from build123d import *

# Parameters (mm, degrees)
SKETCH_1_W          = 6.3
SKETCH_1_H          = 11.9
SKETCH_1_W_2        = 3
SKETCH_1_H_2        = 1.2
EXTRUDE_2_DEPTH     = 3
SKETCH_7_W          = 6.3
SKETCH_7_H          = 5.7
EXTRUDE_4_DEPTH     = 2.8
SKETCH_8_W          = 6.3
SKETCH_8_H          = 6.2
EXTRUDE_5_DEPTH     = 5.2
SKETCH_5_R          = 2.7
SKETCH_5_R_2        = 2.95
CUT_EXTRUDE_3_DEPTH = 15.790960077
FILLET_1_R          = 3


with BuildPart() as part:
    # ｽｹｯﾁ1 → ﾎﾞｽ - 押し出し2 (new body)
    with BuildSketch(Plane.YZ):
        with Locations((0, 5.95)):
            Rectangle(SKETCH_1_W, SKETCH_1_H)
        with Locations((0, -0.6)):
            Rectangle(SKETCH_1_W_2, SKETCH_1_H_2)
    extrude(amount=-EXTRUDE_2_DEPTH)

    # ｽｹｯﾁ7 → ﾎﾞｽ - 押し出し4 (add)
    with BuildSketch(Plane(origin=(-3, 0, 0), x_dir=(0, -1, 0), z_dir=(-1, 0, 0))):
        with Locations((0, 2.85)):
            Rectangle(SKETCH_7_W, SKETCH_7_H)
    extrude(amount=EXTRUDE_4_DEPTH)

    # ｽｹｯﾁ8 → ﾎﾞｽ - 押し出し5 (add)
    with BuildSketch(Plane(origin=(-3, 0, 0), x_dir=(0, -1, 0), z_dir=(-1, 0, 0))):
        with Locations((0, 8.8)):
            Rectangle(SKETCH_8_W, SKETCH_8_H)
    extrude(amount=EXTRUDE_5_DEPTH)

    # ｽｹｯﾁ5 → ｶｯﾄ - 押し出し3 (cut, through all)
    with BuildSketch(Plane.YZ):
        with Locations(Location((0, 2.9, 0), (0, 0, 270))):
            Circle(SKETCH_5_R)
        with Locations(Location((0, 8.75, 0), (0, 0, 270))):
            Circle(SKETCH_5_R_2)
    extrude(amount=-CUT_EXTRUDE_3_DEPTH, mode=Mode.SUBTRACT)

    # ﾌｨﾚｯﾄ1
    fillet_1_edges = [part.edges().sort_by_distance(p)[0] for p in [
        (-4.1, -3.15, 11.9),
        (-4.1, 3.15, 11.9),
    ]]
    fillet(fillet_1_edges, radius=FILLET_1_R)


solid = part.part
Check sheet for the modelled part. Datum: model origin and axes. Units: mm. A direction names the side the tool comes from. Give positions to 0.01 mm unless a question says otherwise; leave off trailing zeros. Loops run counter-clockwise (first coordinate to the right, second up) from the corner with the lowest first, then second, coordinate; pieces in that order, holes last. Notation, with made-up numbers: M -30,8 L -24,8 A18 ccw -24,37 Z; hole C 84,75 d3. An arc over 180 degrees is marked long. Use a Markdown table: item, result. Add a question column.
Q1. Tool access check on faces 5 (the flat face through (-1, -1.5, -1)), 6 (the flat face through (-3, 0, -1)), 7 (the flat face through (-3, 3.15, 4)), 8 (the flat face through (-1, 1.5, -1)), 9 (the cylindrical face through (-4.04, -2.25, 11.04)). Record the directions out of +Z, -Z, +X, -X, +Y, -Y that give a thin tool (end or side, any length) a straight path to the whole face; none if there is none.
Q2. Sectioned sample at A-A, the plane y = 0. Record the cut outline in (x, z), then the cut area to 3 significant figures.
Q3. Sectioned sample at B-B, the plane x = -2.75. Record the cut outline in (y, z), then the cut area to 3 significant figures.
Q4. Sectioned sample at D-D, the plane x = -7.5. Record the cut outline in (y, z), then the cut area to 3 significant figures.
Q5. Go/stop test with a flat-tipped pin: pin 1 (0.7 mm diameter, centred on x = -7, y = 1, fed in from -Z). Record where the tip stops, or that it passes through.
Q6. Mould release check, pull along Y, two halves, no side actions. Record for faces 1 (the cylindrical face through (-4, 0.1, 11.7)), 2 (the flat face through (-1, 0, -1.2)), 3 (the cylindrical face through (-2.859, -1.643, 5.043)), 4 (the flat face through (-3, -3.15, 4)): pulls with the +Y half, pulls with the -Y half, needs draft (parallel to the pull), parting line crosses it, or undercut.
Q7. Scan lines: line 1 along Z through (x, y) = (-5.5, -0.75); line 2 along Y through (x, z) = (-2.45, 2.9); line 3 along Y through (x, z) = (-5.5, 8.75). Record each from-to range of solid material in increasing order. Write a range as [from, to].
Q8. Sectioned sample at C-C, the plane z = 2.9. Record the cut outline in (x, y), then the cut area to 3 significant figures.
Verdict:
| question | item | result |
|---|---|---|
| 1 | face 5 | -Z, +X, -X, -Y |
| 1 | face 6 | -Z, -X, +Y, -Y |
| 1 | face 7 | +Z, -Z, +X, -X, +Y |
| 1 | face 8 | -Z, +X, -X, +Y |
| 1 | face 9 | +Z, +X, -X, -Y |
| 2 | outline | M -8.2,5.7 L -5.8,5.7 L -5.8,5.6 L 0,5.6 L 0,5.8 L -8.2,5.8 Z; M -8.2,11.7 L 0,11.7 L 0,11.9 L -8.2,11.9 Z; M -5.8,0 L -3,0 L -3,-1.2 L 0,-1.2 L 0,0.2 L -5.8,0.2 Z |
| 2 | area | 7.80 mm^2 |
| 3 | outline | M -3.15,0 L -1.5,0 L -1.5,-1.2 L 1.5,-1.2 L 1.5,0 L 3.15,0 L 3.15,8.9 A3 ccw 0.15,11.9 L -0.15,11.9 A3 ccw -3.15,8.9 Z; hole C 0,8.75 d5.9; hole C 0,2.9 d5.4 |
| 3 | area | 24.5 mm^2 |
| 4 | outline | M -3.15,5.7 L 3.15,5.7 L 3.15,8.9 A3 ccw 0.15,11.9 L -0.15,11.9 A3 ccw -3.15,8.9 Z; hole C 0,8.75 d5.9 |
| 4 | area | 7.86 mm^2 |
| 5 | pin 1 | z = 5.7 |
| 6 | face 1 | undercut |
| 6 | face 2 | needs draft |
| 6 | face 3 | undercut |
| 6 | face 4 | pulls with the -Y half |
| 7 | line 1 | [0, 0.31], [5.49, 5.9], [11.6, 11.84] |
| 7 | line 2 | [-3.15, -2.7], [2.7, 3.15] |
| 7 | line 3 | [-3.15, -2.95], [2.95, 3.15] |
| 8 | outline | M -5.8,-3.15 L 0,-3.15 L 0,-2.7 L -5.8,-2.7 Z; M -5.8,2.7 L 0,2.7 L 0,3.15 L -5.8,3.15 Z |
| 8 | area | 5.22 mm^2 |
